from build123d import *

# Parameters (mm, degrees)
SKETCH1_W           = 12.7
SKETCH1_H           = 25.4
BOSS_EXTRUDE1_DEPTH = 5.0546


with BuildPart() as part:
    # Sketch1 → Revolve1 (revolve)
    with BuildSketch(Plane.XY):
        with Locations((-6.35, 12.7)):
            Rectangle(SKETCH1_W, SKETCH1_H)
    revolve(axis=Axis((0, 0, 0), (0, -1, 0)))

    # Sketch2 → Boss-Extrude1 (add)
    with BuildSketch(Plane.XZ):
        Polygon((0, 13.746380944), (-9.720159182, 9.720159182), (-13.746380944, 0), (-9.720159182, -9.720159182), (0, -13.746380944), (9.720159182, -9.720159182), (13.746380944, 0), (9.720159182, 9.720159182), align=None)
    extrude(amount=-BOSS_EXTRUDE1_DEPTH)

    # Sketch4 → 1/4 NPT Tapped Hole1 (revolve, cut)
    with BuildSketch(Plane(origin=(0, 0, 0), x_dir=(0, 0, -1), z_dir=(1, 0, 0))):
        Polygon((0, 0), (0, 25.4), (5.5626, 25.4), (5.5626, 10.0203), (5.943679799, 10.0203), (6.243701, 0), align=None)
    revolve(axis=Axis((0, -6.35, 0), (0, 1, 0)), mode=Mode.SUBTRACT)


solid = part.part
Input: part model. Units: mm. Frame: model coordinates. A direction names the side the tool comes from. Give positions to 0.01 mm unless a question says otherwise; leave off trailing zeros. Order: outer loops, then holes, each group sorted by start corner. A loop starts at its lowest first (then second) coordinate and runs counter-clockwise, first axis right, second up.
Q1. Ray query, probe 1 along X at (y, z) = (19.5, 0); probe 2 along Z at (x, y) = (-2.75, 23.5). Return the intervals inside material, ascending.
Checked values:
probe 1: x = -12.7 to -5.56, 5.56 to 12.7
probe 2: z = -12.4 to -4.84, 4.84 to 12.4
Q2. Section C-C on x = 11. Output: boundary loops of the cut face in (y, z), and give its area (3 significant figures).
Checked values:
outline: (0, -6.63) - (5.05, -6.63) - (5.05, -6.35) - (25.4, -6.35) - (25.4, 6.35) - (5.05, 6.35) - (5.05, 6.63) - (0, 6.63) - close
area: 325 mm2
Q3. Section A-A on y = 2. Output: boundary loops of the cut face in (x, z).
Checked values:
outline: (-13.75, 0) - (-9.72, -9.72) - (0, -13.75) - (9.72, -9.72) - (13.75, 0) - (9.72, 9.72) - (0, 13.75) - (-9.72, 9.72) - close; hole circle Ø12.37 at (0, 0)
Q4. Draft query along Z for faces 1 (the flat face through (-9.1, 5.055, 9.1)), 2 (the cylindrical face through (-1.671, 17.602, -5.306)), 3 (the flat face through (-4.928, 2.492, -11.705)). Return one class per face: +Z half, -Z half, draft (parallel to the pull), parting line (faces both ways), or undercut.
Checked values:
face 1: draft
face 2: undercut
face 3: -Z half
Q5. Set-up query: faces 4 (the flat face through (9.3, 5.055, 9.1)), 5 (the flat face through (6, 0, -3)), 6 (the conical face through (-6.044, 4.94, 0.794)), 7 (the flat face through (0, 5.055, -13)). Return all of +Z, -Z, +X, -X, +Y, -Y with unobstructed straight access to the full face (end or side cutting, diameter ignored); none if empty.
Checked values:
face 4: +Z, +X, +Y
face 5: +Z, -Z, +X, -X, -Y
face 6: -Y
face 7: -Z, +Y
Q6. Section D-D on y = 14.5. Output: boundary loops of the cut face in (x, z), and give its area (3 significant figures).
Checked values:
outline: circle Ø25.4 at (0, 0); hole circle Ø11.13 at (0, 0)
area: 409 mm2
Q7. Section B-B on z = 7.75. Output: boundary loops of the cut face in (x, y).
Checked values:
outline: (-10.54, 0) - (10.54, 0) - (10.54, 5.05) - (10.06, 5.05) - (10.06, 25.4) - (-10.06, 25.4) - (-10.06, 5.05) - (-10.54, 5.05) - close
Q8. Contact query for flat-ended pins moving along their axis: pin 1 Ø1.5 at (x, y) = (-1.5, 15.5) entering from -Z; pin 2 Ø4 at (y, z) = (17.5, -8) entering from +X; pin 3 Ø2 at (y, z) = (14, 3) entering from -X; pin 4 Ø10 at (x, z) = (0, 0) entering from -Y. Output: stop coordinate, or through.
Checked values:
pin 1: stops at z = -12.68
pin 2: stops at x = 11.19
pin 3: stops at x = -12.54
pin 4: passes through
